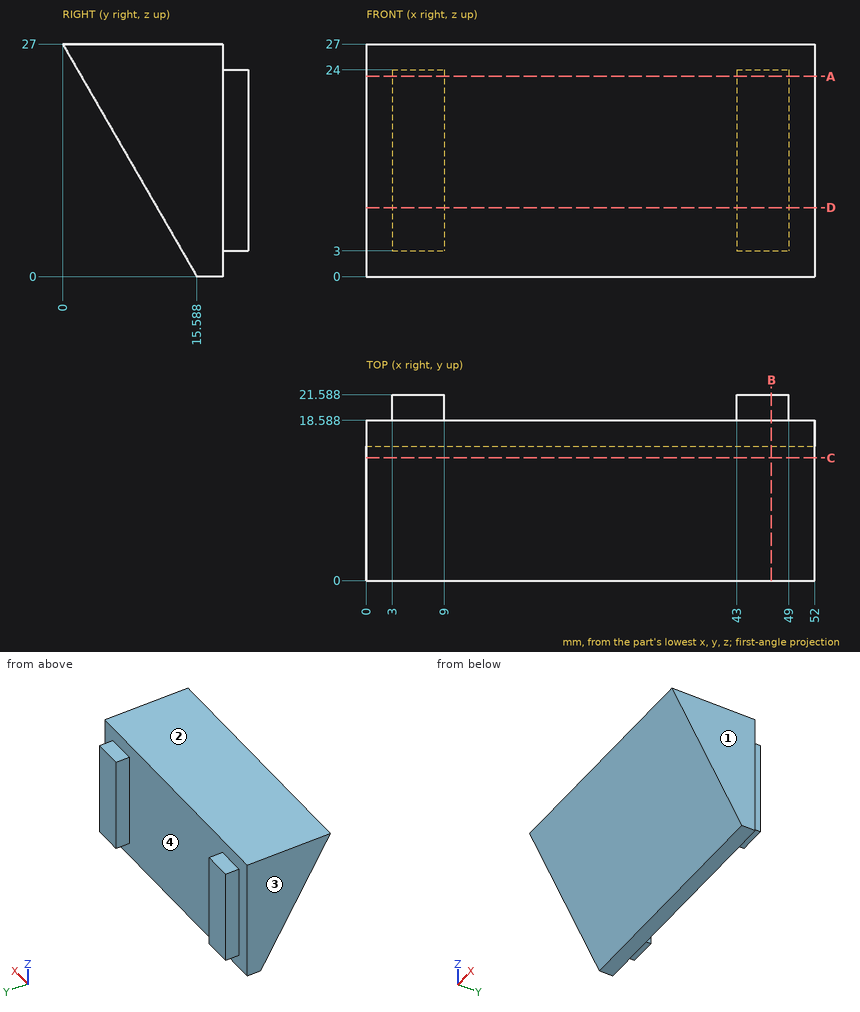
Could you check a few things on this drawing? It's one solid part, dimensions in mm from its lowest x, y, z. Coordinates: 2 decimals unless noted, no trailing zeros. Loops run counter-clockwise (first coordinate to the right, second up) from the corner with the lowest first, then second, coordinate; pieces in that order, holes last.
1. For P1, Ø2.5, axis at y = 20, z = 16.5, coming from the -X side; P2, Ø2.5, axis at x = 6, y = 19.5, coming from the +Z side; P3, Ø1.5, axis at y = 19.5, z = 13.5, coming from the +X side; P4, Ø1.5, axis at x = 4.5, y = 19.5, coming from the -Z side, each with a flat end and sliding along its axis, tell me the tip position at first contact or that it passes through.
2. I need wall thicknesses on L1, parallel to X at y = 20.5, z = 4; L2, parallel to Z at x = 34.5, y = 13.25; L3, parallel to Y at x = 22, z = 20.5. Which ranges of each line are inside material? Lowest first, please.
3. Imagine slicing it at C-C (y = 14.25). Please give me the cut outline in (x, z).
4. Imagine slicing it at D-D (z = 8). Please give me the cut outline in (x, y), and give its area (3 significant figures).
5. We'd pull the mould along X, two halves only. Please class the marked faces 1, 2, 3 and 4: released by +X, released by -X, zero draft, split by the parting line, or undercut.
6. Imagine slicing it at A-A (z = 23.25). Please give me the cut outline in (x, y) (1 decimal).
7. Imagine slicing it at B-B (x = 47). Please give me the cut outline in (y, z).
Computed values:
1. P1: stops at x = 3
1. P2: stops at z = 27
1. P3: stops at x = 49
1. P4: stops at z = 3
2. L1: x = 3 to 9, 43 to 49
2. L2: z = 4.05 to 27
2. L3: y = 3.75 to 18.59
3. outline: (0, 2.32) - (52, 2.32) - (52, 27) - (0, 27) - close
4. outline: (0, 10.97) - (52, 10.97) - (52, 18.59) - (49, 18.59) - (49, 21.59) - (43, 21.59) - (43, 18.59) - (9, 18.59) - (9, 21.59) - (3, 21.59) - (3, 18.59) - (0, 18.59) - close
4. area: 432 mm2
5. face 1: released by +X
5. face 2: zero draft
5. face 3: released by -X
5. face 4: undercut
6. outline: (0, 2.2) - (52, 2.2) - (52, 18.6) - (49, 18.6) - (49, 21.6) - (43, 21.6) - (43, 18.6) - (9, 18.6) - (9, 21.6) - (3, 21.6) - (3, 18.6) - (0, 18.6) - close
7. outline: (0, 27) - (15.59, 0) - (18.59, 0) - (18.59, 3) - (21.59, 3) - (21.59, 24) - (18.59, 24) - (18.59, 27) - close
